Input: part model. Units: mm. Frame: model coordinates. Face numbers are marked on the shaded views. A direction names the side the tool comes from. Round coordinates to 2 decimals unless told otherwise and drop trailing zeros. Loops run counter-clockwise (first coordinate to the right, second up) from the corner with the lowest first, then second, coordinate; pieces in that order, holes last. Notation, with made-up numbers: M -2.75,51.5 L 31.25,51.5 A20 ccw 31.25,71.5 Z; hole C 74.5,-15.75 d6. An arc over 180 degrees is marked long. Return JSON: item names as keys, results as strings. Group by question number.
1) Section C-C (y = -1.4). Output: boundary loops of the cut face in (x, z).
2) Section B-B (z = -41.5). Output: boundary loops of the cut face in (x, y).
3) Access query for the marked faces 1, 2 and 3. Directions: +Z, -Z, +X, -X, +Y, -Y. A direction counts if a zero-diameter tool reaches every point of the face in a straight line with its end or side. Return the directions, or none.
4) Section D-D (x = 16.5). Output: boundary loops of the cut face in (y, z), plus the area to 3 significant figures.
5) Material intervals for line 1 (X direction, y = -1.95, z = -44.75); line 2 (Z direction, x = 23.75, y = -1.3); line 3 (Z direction, x = 14.75, y = -1.1), sorted ascending. Write a range as from..to.
6) Section A-A (x = 24). Output: boundary loops of the cut face in (y, z), plus the area to 3 significant figures.
7) Mould query, pull axis Z, two halves, no side actions, for the marked faces 4, 5 and 6. Classes: +Z half, -Z half, draft (parallel to the pull), parting line (faces both ways), or undercut.
from build123d import *

# Parameters (mm, degrees)
F1_DEPTH     = 3.81
F3_START     = -0.000254
F3_DEPTH     = 3.81
F4_R         = 0.2501042953
F5_DEPTH     = 50.8
F6_T1_DEPTH  = 7.493
F6_T3_DEPTH  = 6.5405
F6_T5_DEPTH  = 7.493
F6_T7_DEPTH  = 6.5405
F6_T9_DEPTH  = 8.636
F6_T11_DEPTH = 10.541
F7_R         = 0.2501042953
F8_DEPTH     = 50.8


# Not quite as in the source:
# - a fillet or chamfer that OpenCascade refuses, or shapes differently, is made with other operations: its cross-section is extruded or revolved along the edge and cut away or added


with BuildPart() as f1:
    # F0 (on Front) → F1 (new body)
    with BuildSketch(Plane.XZ):
        Polygon((23.3729397243, -34.7344989846), (17.0229397243, -34.7344989846), (13.2129397243, -34.7344989846), (13.2129397243, -43.3704989846), (17.0229397243, -43.3704989846), (23.3729397243, -43.3704989846), align=None)
    extrude(amount=F1_DEPTH)

    # F2 (on face) → F3 (join)
    with BuildSketch(Plane.XZ.offset(3.81).offset(F3_START)):
        Polygon((27.1829397243, -29.1464989846), (17.0229397243, -29.1464989846), (17.0229397243, -34.7344989846), (23.3729397243, -34.7344989846), (27.1829397243, -34.7344989846), align=None)
        Polygon((27.1829397243, -43.3704989846), (23.3729397243, -43.3704989846), (17.0229397243, -43.3704989846), (17.0229397243, -48.9584989846), (27.1829397243, -48.9584989846), align=None)
    extrude(amount=-F3_DEPTH)

    # F4 (on face) → F5 (cut)
    with BuildSketch(Plane(origin=(0, 0, -48.9584989846), x_dir=(1, 0, 0), z_dir=(0, 0, -1))):
        with Locations((26.094635429, 1.904746)):
            Circle(F4_R)
    extrude(amount=-F5_DEPTH, mode=Mode.SUBTRACT)

    # F6: fillet of radius 0.381 on 12 edges, made by hand

    # F6_s2 → F6_t1 (cut)
    with BuildSketch(Plane.XY.offset(-35.6869989846)):
        with BuildLine():
            ThreePointArc((26.8019397243, -3.809746), (27.071347408, -3.6981536836), (27.1829397243, -3.428746))
            Line((27.1829397243, -3.428746), (27.1829397243, -3.809746))
            Line((27.1829397243, -3.809746), (26.8019397243, -3.809746))
        make_face()
        with BuildLine():
            ThreePointArc((27.1829397243, -0.380746), (27.071347408, -0.1113383164), (26.8019397243, 0.000254))
            Line((26.8019397243, 0.000254), (27.1829397243, 0.000254))
            Line((27.1829397243, 0.000254), (27.1829397243, -0.380746))
        make_face()
    extrude(amount=F6_T1_DEPTH, mode=Mode.SUBTRACT)

    # F6_s4 → F6_t3 (cut)
    with BuildSketch(Plane.XY.offset(-34.7344989846)):
        with BuildLine():
            ThreePointArc((17.4039397243, -3.809746), (17.1345320407, -3.6981536836), (17.0229397243, -3.428746))
            Line((17.0229397243, -3.428746), (17.0229397243, -3.809746))
            Line((17.0229397243, -3.809746), (17.4039397243, -3.809746))
        make_face()
        with BuildLine():
            ThreePointArc((17.0229397243, -0.380746), (17.1345320407, -0.1113383164), (17.4039397243, 0.000254))
            Line((17.4039397243, 0.000254), (17.0229397243, 0.000254))
            Line((17.0229397243, 0.000254), (17.0229397243, -0.380746))
        make_face()
    extrude(amount=F6_T3_DEPTH, mode=Mode.SUBTRACT)

    # F6_s6 → F6_t5 (cut)
    with BuildSketch(Plane.XY.offset(-49.9109989846)):
        with BuildLine():
            ThreePointArc((26.8019397243, -3.809746), (27.071347408, -3.6981536836), (27.1829397243, -3.428746))
            Line((27.1829397243, -3.428746), (27.1829397243, -3.809746))
            Line((27.1829397243, -3.809746), (26.8019397243, -3.809746))
        make_face()
        with BuildLine():
            ThreePointArc((27.1829397243, -0.380746), (27.071347408, -0.1113383164), (26.8019397243, 0.000254))
            Line((26.8019397243, 0.000254), (27.1829397243, 0.000254))
            Line((27.1829397243, 0.000254), (27.1829397243, -0.380746))
        make_face()
    extrude(amount=F6_T5_DEPTH, mode=Mode.SUBTRACT)

    # F6_s8 → F6_t7 (cut)
    with BuildSketch(Plane.XY.offset(-49.9109989846)):
        with BuildLine():
            ThreePointArc((17.0229397243, -3.428746), (17.1345320407, -3.6981536836), (17.4039397243, -3.809746))
            Line((17.4039397243, -3.809746), (17.0229397243, -3.809746))
            Line((17.0229397243, -3.809746), (17.0229397243, -3.428746))
        make_face()
        with BuildLine():
            ThreePointArc((17.0229397243, -0.380746), (17.1345320407, -0.1113383164), (17.4039397243, 0.000254))
            Line((17.4039397243, 0.000254), (17.0229397243, 0.000254))
            Line((17.0229397243, 0.000254), (17.0229397243, -0.380746))
        make_face()
    extrude(amount=F6_T7_DEPTH, mode=Mode.SUBTRACT)

    # F6_s10 → F6_t9 (cut)
    with BuildSketch(Plane.XY.offset(-43.3704989846)):
        with BuildLine():
            ThreePointArc((22.9919397243, -3.81), (23.261347408, -3.6984076836), (23.3729397243, -3.429))
            Line((23.3729397243, -3.429), (23.3729397243, -3.81))
            Line((23.3729397243, -3.81), (22.9919397243, -3.81))
        make_face()
        with BuildLine():
            ThreePointArc((22.9919397243, 0), (23.261347408, -0.1115923164), (23.3729397243, -0.381))
            Line((23.3729397243, -0.381), (23.3729397243, 0))
            Line((23.3729397243, 0), (22.9919397243, 0))
        make_face()
    extrude(amount=F6_T9_DEPTH, mode=Mode.SUBTRACT)

    # F6_s12 → F6_t11 (cut)
    with BuildSketch(Plane.XY.offset(-44.3229989846)):
        with BuildLine():
            ThreePointArc((13.2129397243, -3.429), (13.3245320407, -3.6984076836), (13.5939397243, -3.81))
            Line((13.5939397243, -3.81), (13.2129397243, -3.81))
            Line((13.2129397243, -3.81), (13.2129397243, -3.429))
        make_face()
        with BuildLine():
            ThreePointArc((13.5939397243, 0), (13.3245320407, -0.1115923164), (13.2129397243, -0.381))
            Line((13.2129397243, -0.381), (13.2129397243, 0))
            Line((13.2129397243, 0), (13.5939397243, 0))
        make_face()
    extrude(amount=F6_T11_DEPTH, mode=Mode.SUBTRACT)

    # F7 (on face) → F8 (cut)
    with BuildSketch(Plane(origin=(0, 0, -43.3704989846), x_dir=(1, 0, 0), z_dir=(0, 0, -1))):
        with Locations((15.1179397243, 1.904746)):
            Circle(F7_R)
    extrude(amount=-F8_DEPTH, mode=Mode.SUBTRACT)


solid = f1.part
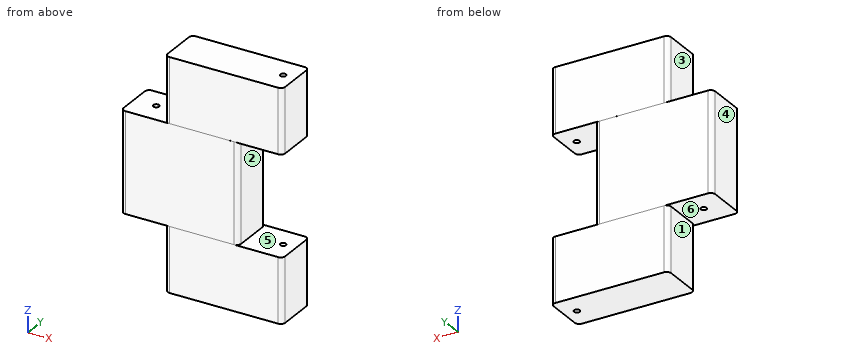
Returned:
{
 "1": {"outline": "M 13.21,-43.37 L 17.02,-43.37 L 17.02,-48.96 L 27.18,-48.96 L 27.18,-43.37 L 23.37,-43.37 L 23.37,-34.73 L 27.18,-34.73 L 27.18,-29.15 L 17.02,-29.15 L 17.02,-34.73 L 13.21,-34.73 Z"},
 "2": {"outline": "M 13.21,-3.43 A0.38 ccw 13.59,-3.81 L 22.99,-3.81 A0.38 ccw 23.37,-3.43 L 23.37,-0.38 A0.38 ccw 22.99,0 L 13.59,0 A0.38 ccw 13.21,-0.38 Z; hole C 15.12,-1.9 d0.5"},
 "3": {"face 1": "-Z, -X, +Y, -Y", "face 2": "+X, +Y, -Y", "face 3": "+Z, -X, +Y, -Y"},
 "4": {"outline": "M -3.81,-43.37 L 0,-43.37 L 0,-34.73 L -3.81,-34.73 Z", "area": "32.9 mm^2"},
 "5": {"line 1": "x = 17.02..25.85, 26.34..27.18", "line 2": "z = -48.96..-43.37, -34.73..-29.15", "line 3": "z = -43.37..-34.73"},
 "6": {"outline": "M -3.81,-48.96 L 0,-48.96 L 0,-43.37 L -3.81,-43.37 Z; M -3.81,-34.73 L 0,-34.73 L 0,-29.15 L -3.81,-29.15 Z", "area": "42.6 mm^2"},
 "7": {"face 4": "draft", "face 5": "undercut", "face 6": "-Z half"}
}
